Geometry check sheet. Reference: drawing and pictorial views, mm from the part's lowest x, y, z. Give positions to 0.01 mm unless a question says otherwise; leave off trailing zeros. Write each loop counter-clockwise with the first axis right and the second up, starting at its lowest first coordinate (ties: lowest second). Pieces come first, ordered by that corner, then holes.
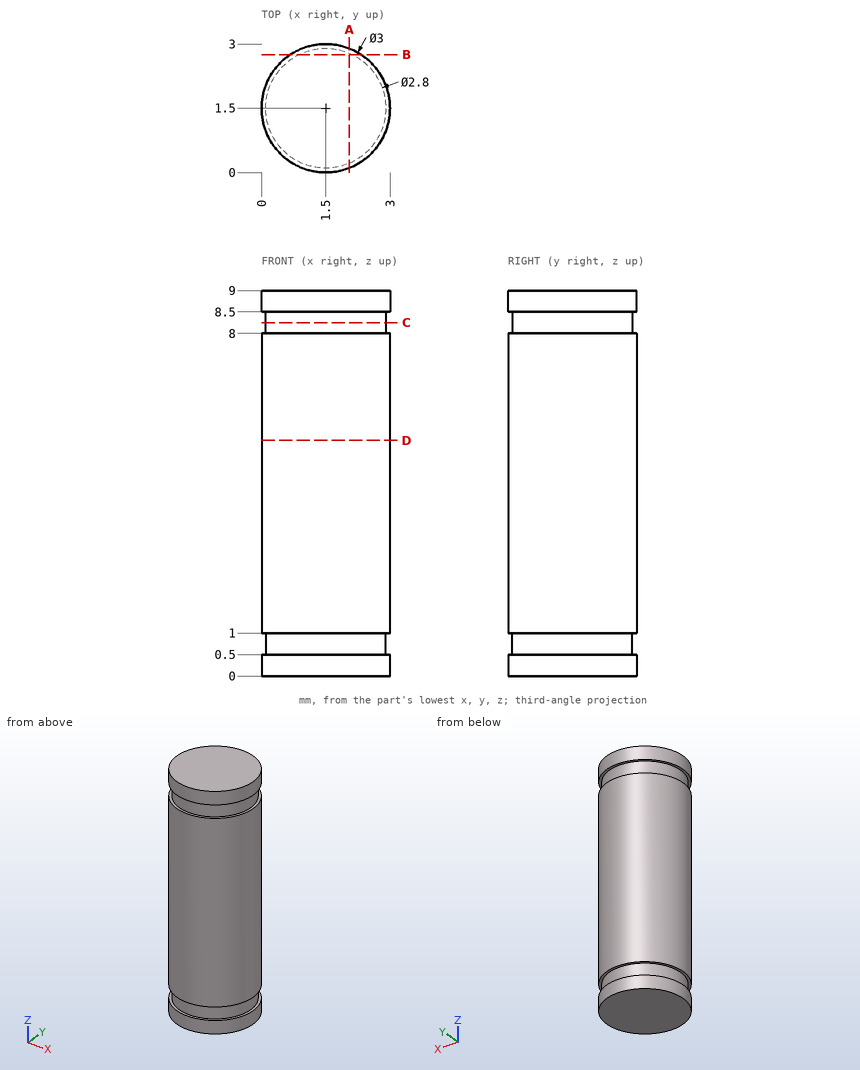
Item 1: Depth check by flat-ended pin: pin 1 (1.5 mm diameter, centred on y = 0.5, z = 4.5, fed in from -X). Enter the tip coordinate at first touch or a pass-through.
Answer key:
pin 1: stops at x = 0.02
Item 2: Sectioned sample at B-B on y = 2.75. Record the cut outline in (x, z).
Answer key:
outline: (0.67, 0) - (2.33, 0) - (2.33, 0.5) - (2.13, 0.5) - (2.13, 1) - (2.33, 1) - (2.33, 8) - (2.13, 8) - (2.13, 8.5) - (2.33, 8.5) - (2.33, 9) - (0.67, 9) - (0.67, 8.5) - (0.87, 8.5) - (0.87, 8) - (0.67, 8) - (0.67, 1) - (0.87, 1) - (0.87, 0.5) - (0.67, 0.5) - close
Item 3: Sectioned sample at C-C on z = 8.25. Record the cut outline in (x, y).
Answer key:
outline: circle Ø2.8 at (1.5, 1.5)
Item 4: Scan lines: line 1 along Y through (x, z) = (0.3, 6); line 2 along Y through (x, z) = (1.4, 7.5); line 3 along X through (y, z) = (2.55, 3.5). Record each from-to range of solid material in increasing order.
Answer key:
line 1: y = 0.6 to 2.4
line 2: y = 0 to 3
line 3: x = 0.43 to 2.57
Item 5: Sectioned sample at D-D on z = 5.5. Record the cut outline in (x, y), then the cut area to 3 significant figures.
Answer key:
outline: circle Ø3 at (1.5, 1.5)
area: 7.07 mm2
Item 6: Sectioned sample at A-A on x = 2.05. Record the cut outline in (y, z).
Answer key:
outline: (0.1, 0) - (2.9, 0) - (2.9, 0.5) - (2.79, 0.5) - (2.79, 1) - (2.9, 1) - (2.9, 8) - (2.79, 8) - (2.79, 8.5) - (2.9, 8.5) - (2.9, 9) - (0.1, 9) - (0.1, 8.5) - (0.21, 8.5) - (0.21, 8) - (0.1, 8) - (0.1, 1) - (0.21, 1) - (0.21, 0.5) - (0.1, 0.5) - close
